```python
from build123d import *

# Parameters (mm, degrees)
SKETCH8_W           = 200
SKETCH8_H           = 60
BOSS_EXTRUDE6_DEPTH = 6
SKETCH9_W           = 60
SKETCH9_H           = 10
BOSS_EXTRUDE7_DEPTH = 50
SKETCH10_R          = 2
SKETCH10_W          = 41
SKETCH10_H          = 20
CUT_EXTRUDE8_DEPTH  = 10
SKETCH15_W          = 58
SKETCH15_H          = 28
BOSS_EXTRUDE9_DEPTH = 7
SKETCH12_W          = 51
SKETCH12_H          = 21
CUT_EXTRUDE9_DEPTH  = 7
SKETCH13_R          = 3
CUT_EXTRUDE10_DEPTH = 2
SKETCH17_R          = 1.65
CUT_EXTRUDE11_DEPTH = 4
FILLET1_R           = 1.5
FILLET2_R           = 1.5


with BuildPart() as part:
    # Sketch8 → Boss-Extrude6 (new body)
    with BuildSketch(Plane(origin=(0, 0, 0), x_dir=(1, 0, 0), z_dir=(0, 1, 0))):
        Rectangle(SKETCH8_W, SKETCH8_H)
    extrude(amount=BOSS_EXTRUDE6_DEPTH)

    # Sketch9 → Boss-Extrude7 (add)
    with BuildSketch(Plane(origin=(0, 6, 0), x_dir=(1, 0, 0), z_dir=(0, 1, 0))):
        with Locations((70, 25)):
            Rectangle(SKETCH9_W, SKETCH9_H)
    extrude(amount=BOSS_EXTRUDE7_DEPTH)

    # Sketch10 → Cut-Extrude8 (cut)
    with BuildSketch(Plane.XY.offset(-20)):
        with Locations((45.75, 51)):
            Circle(SKETCH10_R)
        with Locations((45.75, 41)):
            Circle(SKETCH10_R)
        with Locations((70, 46)):
            Rectangle(SKETCH10_W, SKETCH10_H)
        with Locations((94.25, 51)):
            Circle(SKETCH10_R)
        with Locations((94.25, 41)):
            Circle(SKETCH10_R)
    extrude(amount=-CUT_EXTRUDE8_DEPTH, mode=Mode.SUBTRACT)

    # Sketch15 → Boss-Extrude9 (add)
    with BuildSketch(Plane(origin=(0, 6, 0), x_dir=(1, 0, 0), z_dir=(0, 1, 0))):
        with Locations((0, -6.66875)):
            Rectangle(SKETCH15_W, SKETCH15_H)
    extrude(amount=BOSS_EXTRUDE9_DEPTH)

    # Sketch12 → Cut-Extrude9 (cut)
    with BuildSketch(Plane(origin=(0, 13, 0), x_dir=(1, 0, 0), z_dir=(0, 1, 0))):
        with Locations((0, -6.66875)):
            Rectangle(SKETCH12_W, SKETCH12_H)
    extrude(amount=-CUT_EXTRUDE9_DEPTH, mode=Mode.SUBTRACT)

    # Sketch13 → Cut-Extrude10 (cut)
    with BuildSketch(Plane(origin=(0, 0, 0), x_dir=(-1, 0, 0), z_dir=(0, -1, 0))):
        with Locations(Location((-15.5, -2.16875, 0), (0, 0, 90))):
            Circle(SKETCH13_R)
        with Locations(Location((-15.5, -11.16875, 0), (0, 0, 90))):
            Circle(SKETCH13_R)
        with Locations(Location((15.5, -2.16875, 0), (0, 0, 90))):
            Circle(SKETCH13_R)
        with Locations(Location((15.5, -11.16875, 0), (0, 0, 90))):
            Circle(SKETCH13_R)
    extrude(amount=-CUT_EXTRUDE10_DEPTH, mode=Mode.SUBTRACT)

    # Sketch17 → Cut-Extrude11 (cut)
    with BuildSketch(Plane.XZ.offset(-2)):
        with Locations(Location((-15.5, 11.16875, 0), (0, 0, 270))):
            Circle(SKETCH17_R)
        with Locations(Location((-15.5, 2.16875, 0), (0, 0, 270))):
            Circle(SKETCH17_R)
        with Locations(Location((15.5, 11.16875, 0), (0, 0, 270))):
            Circle(SKETCH17_R)
        with Locations(Location((15.5, 2.16875, 0), (0, 0, 270))):
            Circle(SKETCH17_R)
    extrude(amount=-CUT_EXTRUDE11_DEPTH, mode=Mode.SUBTRACT)

    # Fillet1
    fillet1_edges = [part.edges().sort_by_distance(p)[0] for p in [
        (-29, 6, 6.66875),
        (0, 6, 20.66875),
        (29, 6, 6.66875),
        (0, 6, -7.33125),
    ]]
    fillet(fillet1_edges, radius=FILLET1_R)

    # Fillet2
    fillet2_edges = [part.edges().sort_by_distance(p)[0] for p in [
        (-100, 6, 0),
        (-30, 6, -30),
        (0, 6, 30),
        (100, 31, -20),
        (40, 6, -25),
        (40, 31, -30),
        (70, 6, -20),
        (40, 31, -20),
        (100, 56, -25),
        (40, 56, -25),
        (100, 6, 5),
        (100, 28, -30),
    ]]
    fillet(fillet2_edges, radius=FILLET2_R)


solid = part.part
```
Geometry check sheet. Reference: the model listing, model coordinates, mm. A direction names the side the tool comes from. Coordinates: 2 decimals unless noted, no trailing zeros. Loops run counter-clockwise (first coordinate to the right, second up) from the corner with the lowest first, then second, coordinate; pieces in that order, holes last.
Item 1: Sectioned sample at D-D, the plane y = 25. Record the boundary of the cut face in (x, z).
Item 2: Access from +Z, -Z, +X, -X, +Y, -Y to the whole of each face (thin tool, end or side, straight path). Record for faces 1 (the face through (-29, 10, 7)), 2 (the face through (-18.43, 0.99, 2.82)), 3 (the face through (-1, 6, -13)), 4 (the face through (70, 36, -25)).
Item 3: Sectioned sample at B-B, the plane x = 94.25. Record the boundary of the cut face in (y, z), then the cut area to 3 significant figures.
Item 4: Thickness scan on line 1 (Z direction, x = -17, y = 10); line 2 (Y direction, x = 94, z = -23); line 3 (X direction, y = 10, z = 6.5). Record the ranges inside material, lowest first.
Item 5: Go/stop test with flat-tipped pins: pin 1 Ø10 at (y, z) = (43, -19) entering from -X; pin 2 Ø8 at (x, z) = (71, -26.5) entering from +Y; pin 3 Ø7 at (x, z) = (15.5, 11.17) entering from +Y; pin 4 Ø6 at (x, z) = (9.5, 20) entering from -Y. Record where each tip stops, or that it passes through.
Item 6: Release check for a two-part mould opening along Z. For faces 5 (the face through (70, 26, -20)), 6 (the face through (0, 6, 7)), 7 (the face through (96.097, 40.234, -24.93)) record: released by +Z, released by -Z, zero draft, split by the parting line, or undercut.
Item 7: Sectioned sample at A-A, the plane y = 51. Record the boundary of the cut face in (x, z), then the cut area to 3 significant figures.
Item 8: Sectioned sample at C-C, the plane x = 57. Record the boundary of the cut face in (y, z), then the cut area to 3 significant figures.
Check result:
1. outline: (40, -28.5) arc R1.5 ccw to (41.5, -30) - (98.5, -30) arc R1.5 ccw to (100, -28.5) - (100, -21.5) arc R1.5 ccw to (98.5, -20) - (41.5, -20) arc R1.5 ccw to (40, -21.5) - close
2. face 1: +Z, -Z, -X, +Y
2. face 2: -Y
2. face 3: +Y
2. face 4: +Z, -Z, +Y
3. outline: (0, -30) - (39, -30) - (39, -20) - (7.5, -20) arc R1.5 cw to (6, -18.5) - (6, 28.5) arc R1.5 ccw to (4.5, 30) - (0, 30) - close; (43, -30) - (49, -30) - (49, -20) - (43, -20) - close; (53, -30) - (56, -30) - (56, -20) - (53, -20) - close
3. area: 780 mm2
4. line 1: z = -7.33 to -3.83, 17.17 to 20.67
4. line 2: y = 0 to 39.02, 42.98 to 49.02, 52.98 to 56
4. line 3: x = -29 to -25.5, 25.5 to 29
5. pin 1: stops at x = 40
5. pin 2: stops at y = 36
5. pin 3: stops at y = 6
5. pin 4: stops at y = 0
6. face 5: released by +Z
6. face 6: undercut
6. face 7: zero draft
7. outline: (40, -28.5) arc R1.5 ccw to (41.5, -30) - (43.75, -30) - (43.75, -20) - (41.5, -20) arc R1.5 ccw to (40, -21.5) - close; (47.75, -30) - (49.5, -30) - (49.5, -20) - (47.75, -20) - close; (90.5, -30) - (92.25, -30) - (92.25, -20) - (90.5, -20) - close; (96.25, -30) - (98.5, -30) arc R1.5 ccw to (100, -28.5) - (100, -21.5) arc R1.5 ccw to (98.5, -20) - (96.25, -20) - close
7. area: 108 mm2
8. outline: (0, -30) - (36, -30) - (36, -20) - (7.5, -20) arc R1.5 cw to (6, -18.5) - (6, 28.5) arc R1.5 ccw to (4.5, 30) - (0, 30) - close
8. area: 660 mm2
